from build123d import *

# Parameters (mm, degrees)
F0_W     = 87.414469
F0_H     = 77.576831
F1_DEPTH = 25.9
F2_R     = 29.572162
F2_R_2   = 24.176686
F3_DEPTH = 25
F4_DEPTH = 41.6
F5_DEPTH = 58.3


with BuildPart() as f1:
    # F0 (on Front) → F1 (new body)
    with BuildSketch(Plane.XZ):
        with Locations((0.983765, 0.562154)):
            Rectangle(F0_W, F0_H)
    extrude(amount=F1_DEPTH)

    # F2 (on face) → F3 (join)
    with BuildSketch(Plane.XZ.offset(25.9)):
        Circle(F2_R)
        Circle(F2_R_2, mode=Mode.SUBTRACT)
    extrude(amount=F3_DEPTH)

    # F2 (on face) → F4 (cut)
    with BuildSketch(Plane.XZ.offset(25.9)):
        Circle(F2_R_2)
    extrude(amount=-F4_DEPTH, mode=Mode.SUBTRACT)

    # F2 (on face) → F5 (cut)
    with BuildSketch(Plane.XZ.offset(25.9)):
        Circle(F2_R_2)
    extrude(amount=-F5_DEPTH, mode=Mode.SUBTRACT)


solid = f1.part
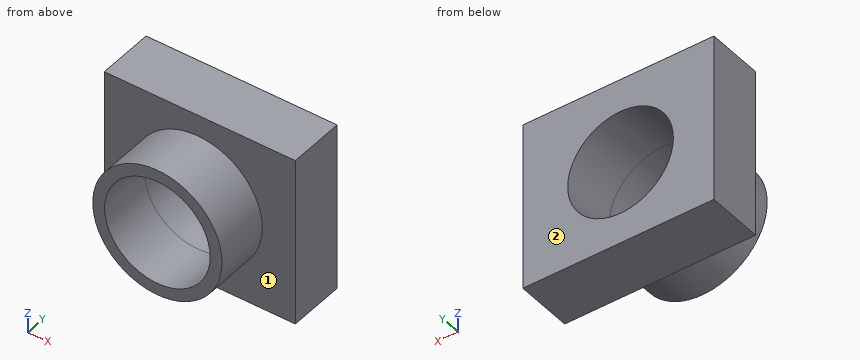
Input: part model. Units: mm. Frame: model coordinates. Face numbers are marked on the shaded views. A direction names the side the tool comes from. Round coordinates to 2 decimals unless told otherwise and drop trailing zeros. Write each loop counter-clockwise with the first axis right and the second up, starting at its lowest first coordinate (ties: lowest second). Pieces come first, ordered by that corner, then holes.
1) Cut plane A-A (z = 0). Return the cut outline in (x, y), then the cut area to 3 significant figures.
2) Ray query, L1, parallel to Z at x = 0, y = -33; L2, parallel to Y at x = 38.5, z = 22.5; L3, parallel to Z at x = -7.5, y = -4. Return the intervals inside material, ascending.
3) Contact query for flat-ended pins moving along their axis: P1, Ø4, axis at x = -23, z = -10.5, coming from the +Y side; P2, Ø1.5, axis at x = 16, y = -42, coming from the +Z side. Output: stop coordinate, or through.
4) Reachability of the marked faces 1 and 2 from +Z, -Z, +X, -X, +Y, -Y: full face, straight path, thin tool, end or side. Return the list, or none.
5) Cut plane B-B (x = -8). Return the cut outline in (y, z).
6) Cut plane D-D (y = -40.5). Return the cut outline in (x, z), then the cut area to 3 significant figures.
7) Cut plane C-C (z = 27.5). Return the cut outline in (x, y).
Geometry says:
1. outline: (-42.72, -25.9) - (-29.57, -25.9) - (-29.57, -50.9) - (-24.18, -50.9) - (-24.18, 0) - (-42.72, 0) - close; (24.18, -50.9) - (29.57, -50.9) - (29.57, -25.9) - (44.69, -25.9) - (44.69, 0) - (24.18, 0) - close
1. area: 1,280 mm2
2. L1: z = -29.57 to -24.18, 24.18 to 29.57
2. L2: y = -25.9 to 0
2. L3: z = -38.23 to -22.98, 22.98 to 39.35
3. P1: stops at y = 0
3. P2: stops at z = 25.34
4. face 1: -Y
4. face 2: +Z, -Z, +X, -X, +Y
5. outline: (-50.9, -28.47) - (-25.9, -28.47) - (-25.9, -38.23) - (0, -38.23) - (0, -22.81) - (-50.9, -22.81) - close; (-50.9, 22.81) - (0, 22.81) - (0, 39.35) - (-25.9, 39.35) - (-25.9, 28.47) - (-50.9, 28.47) - close
6. outline: circle Ø59.14 at (0, 0); hole circle Ø48.35 at (0, 0)
6. area: 911 mm2
7. outline: (-42.72, -25.9) - (-10.87, -25.9) - (-10.87, -50.9) - (10.87, -50.9) - (10.87, -25.9) - (44.69, -25.9) - (44.69, 0) - (-42.72, 0) - close
